from build123d import *

# Parameters (mm, degrees)
F1_DEPTH = 73.025
F2_R     = 6.985
F3_DEPTH = 25.4
F5_W     = 22.225
F5_H     = 36.5125
F6_DEPTH = 25.4


with BuildPart() as f1:
    # F0 (on Front) → F1 (new body)
    with BuildSketch(Plane.XZ):
        Polygon((-17.4625, 0), (-11.1125, 0), (-11.1125, 73.025), (0, 73.025), (0, 79.375), (-17.4625, 79.375), align=None)
    extrude(amount=-F1_DEPTH)

    # F2 (on face) → F3 (cut)
    with BuildSketch(Plane.YZ.offset(-11.1125)):
        with Locations((36.5125, 36.5125)):
            Circle(F2_R)
    extrude(amount=-F3_DEPTH, mode=Mode.SUBTRACT)

    # F4: F1 across plane


with BuildPart() as f1_1:
    add(f1.part)
    add(f1.part.mirror(Plane.YZ))

    # F5 (on face) → F6 (cut)
    with BuildSketch(Plane.XY.offset(79.375)):
        with Locations((0, 18.25625)):
            Rectangle(F5_W, F5_H)
    extrude(amount=-F6_DEPTH, mode=Mode.SUBTRACT)


solid = f1_1.part
Here's how the part is built. I have some questions about the finished solid (model axes, mm). A direction names the side the tool comes from. Give positions to 0.01 mm unless a question says otherwise; leave off trailing zeros. Order: outer loops, then holes, each group sorted by start corner. A loop starts at its lowest first (then second) coordinate and runs counter-clockwise, first axis right, second up. Notation, with made-up numbers: M 71.25,0 L 128.25,0 A5 cw 128.25,7 Z; hole C 2,-31 d2. An arc over 180 degrees is marked long. Answer as a JSON object with one key per item and string values. Group by question number.
1) Please list where these lines run through material, in increasing order: L1, parallel to Z at x = 12, y = 36.5 (3 decimals); L2, parallel to X at y = 31, z = 15; L3, parallel to Z at x = -2, y = 46.5 (3 decimals). Write a range as [from, to].
2) Suppose I cut it at D-D, the plane z = 35.5. Write out the boundary of the cut face in (x, y) (1 decimal), plus the area to 3 significant figures.
3) I'm going to push flat-ended pins straight in: pin 1 Ø12.5 at (y, z) = (36.51, 36.51) entering from -X; pin 2 Ø1.9 at (x, z) = (-1.5, 77.5) entering from -Y; pin 3 Ø6.5 at (x, y) = (4.5, 55.5) entering from -Z (3 decimals). Where does each tip first touch, or does it pass through?
4) Suppose I cut it at A-A, the plane y = 25. Write out the boundary of the cut face in (x, z) (1 decimal).
5) We'd pull the mould along X, two halves only. Please class faces 1 (the cylindrical face through (-14.24, 30.97, 32.26)), 2 (the flat face through (17.462, 44, 40)), 3 (the flat face through (-17.462, 44, 40)), 4 (the flat face through (11.112, 28, 39)): pulls with the +X half, pulls with the -X half, needs draft (parallel to the pull), parting line crosses it, or undercut.
6) On a 3-axis mill with a long thin cutter (end or side, diameter ignored), from which of +Z, -Z, +X, -X, +Y, -Y can I reach the whole of each face in a straight line? I mean faces 5 (the flat face through (14, 0, 40)), 6 (the flat face through (0, 55, 73.025)), 7 (the flat face through (0, 36.512, 76)). Say none if no direction works.
7) Suppose I cut it at C-C, the plane x = 13.5. Write out the boundary of the cut face in (y, z) (1 decimal).
8) Suppose I cut it at B-B, the plane z = 64.5. Write out the boundary of the cut face in (x, y) (1 decimal).
Results found:
{
 "1": {"L1": "[0, 29.528], [43.497, 79.375]", "L2": "[-17.46, -11.11], [11.11, 17.46]", "L3": "[73.025, 79.375]"},
 "2": {"outline": "M -17.5,0 L -11.1,0 L -11.1,29.6 L -17.5,29.6 Z; M -17.5,43.4 L -11.1,43.4 L -11.1,73 L -17.5,73 Z; M 11.1,0 L 17.5,0 L 17.5,29.6 L 11.1,29.6 Z; M 11.1,43.4 L 17.5,43.4 L 17.5,73 L 11.1,73 Z", "area": "752 mm²"},
 "3": {"pin 1": "through", "pin 2": "y = 36.51", "pin 3": "z = 73.025"},
 "4": {"outline": "M -17.5,0 L -11.1,0 L -11.1,79.4 L -17.5,79.4 Z; M 11.1,0 L 17.5,0 L 17.5,79.4 L 11.1,79.4 Z"},
 "5": {"face 1": "needs draft", "face 2": "pulls with the +X half", "face 3": "pulls with the -X half", "face 4": "undercut"},
 "6": {"face 5": "+Z, -Z, +X, -X, -Y", "face 6": "-Z, +Y, -Y", "face 7": "+Z, -Z, -Y"},
 "7": {"outline": "M 0,0 L 73,0 L 73,79.4 L 0,79.4 Z; hole C 36.5,36.5 d14"},
 "8": {"outline": "M -17.5,0 L -11.1,0 L -11.1,73 L -17.5,73 Z; M 11.1,0 L 17.5,0 L 17.5,73 L 11.1,73 Z"}
}
